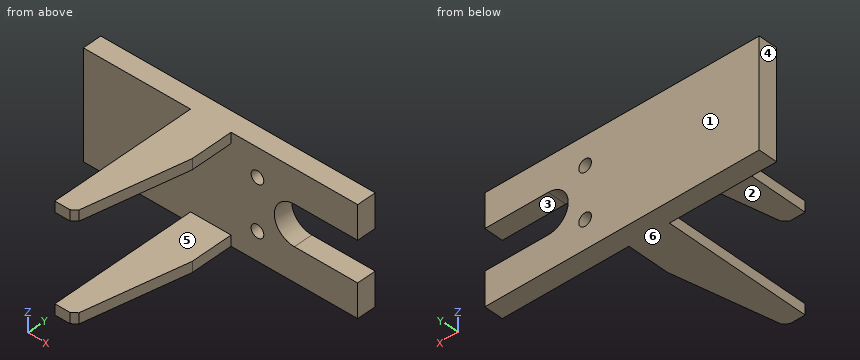
```python
from build123d import *

# Parameters (mm, degrees)
F0_R     = 3
F0_W     = 20
F0_H     = 5
F1_DEPTH = 9
F2_W     = 19.2
F2_H     = 5
F3_DEPTH = 70
F4_SIZE2 = 50
F4_SIZE  = 10
F5_SIZE2 = 50
F5_SIZE  = 10
F6_SIZE  = 2


with BuildPart() as f1:
    # F0 (on Front) → F1 (new body)
    with BuildSketch(Plane.XZ):
        with BuildLine():
            Line((-19.2, 25.4), (-70, 25.4))
            Line((-70, 25.4), (-70, -25.4))
            Line((-70, -25.4), (-19.2, -25.4))
            Line((-19.2, -25.4), (-19.2, -20.4))
            Line((-19.2, -20.4), (0.8, -20.4))
            Line((0.8, -20.4), (0.8, -25.4))
            Line((0.8, -25.4), (60, -25.4))
            Line((60, -25.4), (60, -9.5))
            Line((60, -9.5), (30, -9.5))
            ThreePointArc((30, -9.5), (20.5, 0), (30, 9.5))
            Line((30, 9.5), (60, 9.5))
            Line((60, 9.5), (60, 25.4))
            Line((60, 25.4), (0.8, 25.4))
            Line((0.8, 25.4), (0.8, 20.4))
            Line((0.8, 20.4), (-19.2, 20.4))
            Line((-19.2, 20.4), (-19.2, 25.4))
        make_face()
        with Locations((12.5, -12)):
            Circle(F0_R, mode=Mode.SUBTRACT)
        with Locations((12.5, 12)):
            Circle(F0_R, mode=Mode.SUBTRACT)
        with Locations((-9.2, 22.9)):
            Rectangle(F0_W, F0_H)
        with Locations((-9.2, -22.9)):
            Rectangle(F0_W, F0_H)
    extrude(amount=-F1_DEPTH)

    # F2 (on face) → F3 (join)
    with BuildSketch(Plane.XZ):
        with Locations((-9.6, 22.9)):
            Rectangle(F2_W, F2_H)
        with Locations((-9.6, -22.9)):
            Rectangle(F2_W, F2_H)
    extrude(amount=F3_DEPTH)

    # F4
    f4_edges = [f1.edges().sort_by_distance(p)[0] for p in [
        (0, -70, 22.9),
    ]]
    f4_side = f1.faces().sort_by_distance((-9.6, -70, 22.9))[0]
    chamfer(f4_edges, length=F4_SIZE, length2=F4_SIZE2, reference=f4_side)

    # F5
    f5_edges = [f1.edges().sort_by_distance(p)[0] for p in [
        (0, -70, -22.9),
    ]]
    f5_side = f1.faces().sort_by_distance((-9.6, -70, -22.9))[0]
    chamfer(f5_edges, length=F5_SIZE, length2=F5_SIZE2, reference=f5_side)

    # F6
    f6_edges = [f1.edges().sort_by_distance(p)[0] for p in [
        (-10, -70, 22.9),
        (-10, -70, -22.9),
    ]]
    chamfer(f6_edges, length=F6_SIZE)


solid = f1.part
```
Here's how the part is built. I have some questions about the finished solid (model axes, mm). Face numbers are marked on the shaded views. A direction names the side the tool comes from. Give positions to 0.01 mm unless a question says otherwise; leave off trailing zeros. Loops run counter-clockwise (first coordinate to the right, second up) from the corner with the lowest first, then second, coordinate; pieces in that order, holes last. Notation, with made-up numbers: M 14.25,3 L 20.25,3 A27 cw 20.25,31 Z; hole C -0.75,43 d2. An arc over 180 degrees is marked long. Put each result on its own line as item: value. Start each with the question number.
(1) I need wall thicknesses on line 1 along Z through (x, y) = (12.5, 2.5); line 2 along Z through (x, y) = (-5.5, -22); line 3 along Z through (x, y) = (53, 2). Which ranges of each line are inside material? Lowest first, please. Write a range as [from, to].
(2) Will these pins go through, and if not, where does the flat tip stop? pin 1 Ø12 at (x, z) = (0, -3) entering from -Y; pin 2 Ø4 at (y, z) = (-35.5, -23.5) entering from -X; pin 3 Ø1.5 at (y, z) = (-10, 21.5) entering from +X; pin 4 Ø10 at (x, y) = (-27.5, -32.5) entering from +Z.
(3) I want a section at A-A on y = -14.5. Please give me the cut outline in (x, z).
(4) I want a section at C-C on x = 12.5. Please give me the cut outline in (y, z).
(5) For the marked faces 1, 2 and 3, which set-ups out of +Z, -Z, +X, -X, +Y, -Y let a thin tool reach every point of the face, with its end or its side?
(6) I want a section at D-D on z = 22.5. Please give me the cut outline in (x, y), then the cut area to 3 significant figures.
(7) If we mould it in two halves opening along Z, with no side actions, what happens to the marked faces 4, 5 and 6? For each: +Z half, -Z half, draft (parallel to the pull), parting line (faces both ways), or undercut.
(8) I want a section at B-B on x = 33. Please give me the cut outline in (y, z), then the cut area to 3 significant figures.
Answer block:
1. line 1: [-25.4, -15], [-9, 9], [15, 25.4]
1. line 2: [-25.4, -20.4], [20.4, 25.4]
1. line 3: [-25.4, -9.5], [9.5, 25.4]
2. pin 1: y = 0
2. pin 2: x = -19.2
2. pin 3: x = 0
2. pin 4: through
3. outline: M -19.2,-25.4 L 0,-25.4 L 0,-20.4 L -19.2,-20.4 Z; M -19.2,20.4 L 0,20.4 L 0,25.4 L -19.2,25.4 Z
4. outline: M 0,-25.4 L 9,-25.4 L 9,-15 L 0,-15 Z; M 0,-9 L 9,-9 L 9,9 L 0,9 Z; M 0,15 L 9,15 L 9,25.4 L 0,25.4 Z
5. face 1: +Z, -Z, +X, -X, +Y
5. face 2: +X, -X, -Y
5. face 3: +X, +Y, -Y
6. outline: M -70,0 L -19.2,0 L -19.2,-70 L -12,-70 L -9.61,-68.04 L 0,-20 L 0,0 L 60,0 L 60,9 L -70,9 Z
6. area: 2,260 mm^2
7. face 4: draft
7. face 5: undercut
7. face 6: -Z half
8. outline: M 0,-25.4 L 9,-25.4 L 9,-9.5 L 0,-9.5 Z; M 0,9.5 L 9,9.5 L 9,25.4 L 0,25.4 Z
8. area: 286 mm^2
